```python
from build123d import *

# Parameters (mm, degrees)
SKETCH2_R           = 1.425
BOSS_EXTRUDE1_DEPTH = 3.175


with BuildPart() as part:
    # Sketch2 → Boss-Extrude1 (new body)
    with BuildSketch(Plane(origin=(0, 0, 0), x_dir=(1, 0, 0), z_dir=(0, 1, 0))):
        with BuildLine():
            Line((-145.18277075, -44.880968233), (-179.497120097, -25.768390824))
            ThreePointArc((-179.497120097, -25.768390824), (-183.588653035, -24.128556812), (-187.960968922, -23.569494069))
            Line((-187.960968922, -23.569494069), (-247.377604545, -27.068041697))
            ThreePointArc((-247.377604545, -27.068041697), (-255.760524502, -29.218913898), (-262.07032604, -35.142257782))
            ThreePointArc((-262.07032604, -35.142257782), (-266.807761783, -43.251676507), (-270.933745897, -51.688632391))
            Line((-270.933745897, -51.688632391), (-273.728235609, -57.981701498))
            ThreePointArc((-273.728235609, -57.981701498), (-274.847170355, -61.434035543), (-275.2256366, -65.043382939))
            Line((-275.2256366, -65.043382939), (-275.2256366, -88.130010281))
            ThreePointArc((-275.2256366, -88.130010281), (-270.129294593, -100.433668273), (-257.8256366, -105.530010281))
            Line((-257.8256366, -105.530010281), (-193.494425739, -105.530010281))
            ThreePointArc((-193.494425739, -105.530010281), (-186.835734016, -104.205514146), (-181.190767747, -100.433668273))
            Line((-181.190767747, -100.433668273), (-180.680815133, -99.923715659))
            ThreePointArc((-180.680815133, -99.923715659), (-176.755292612, -97.300765368), (-172.12482308, -96.379707712))
            Line((-172.12482308, -96.379707712), (-153.649556898, -96.379707712))
            ThreePointArc((-153.649556898, -96.379707712), (-141.345898905, -91.283365704), (-136.249556898, -78.979707712))
            Line((-136.249556898, -78.979707712), (-136.249556898, -73.280889471))
            Line((-136.249556898, -73.280889471), (-138.999556898, -73.280889471))
            Line((-138.999556898, -73.280889471), (-138.999556898, -65.780889471))
            Line((-138.999556898, -65.780889471), (-136.249556898, -65.780889471))
            Line((-136.249556898, -65.780889471), (-136.249556898, -60.08207123))
            ThreePointArc((-136.249556898, -60.08207123), (-138.648188978, -51.266235449), (-145.18277075, -44.880968233))
        make_face()
        with Locations(Location((-147.207602145, -91.127288498, 0), (0, 0, 270))):
            Circle(SKETCH2_R, mode=Mode.SUBTRACT)
        with Locations(Location((-141.795027651, -53.115534334, 0), (0, 0, 270))):
            Circle(SKETCH2_R, mode=Mode.SUBTRACT)
        with Locations(Location((-187.963906245, -27.219493821, 0), (0, 0, 270))):
            Circle(SKETCH2_R, mode=Mode.SUBTRACT)
        with Locations(Location((-253.051529835, -31.941972813, 0), (0, 0, 270))):
            Circle(SKETCH2_R, mode=Mode.SUBTRACT)
        with Locations(Location((-267.548354841, -97.852728522, 0), (0, 0, 270))):
            Circle(SKETCH2_R, mode=Mode.SUBTRACT)
        with Locations(Location((-202.85468144, -101.880010281, 0), (0, 0, 270))):
            Circle(SKETCH2_R, mode=Mode.SUBTRACT)
    extrude(amount=BOSS_EXTRUDE1_DEPTH)


solid = part.part
```
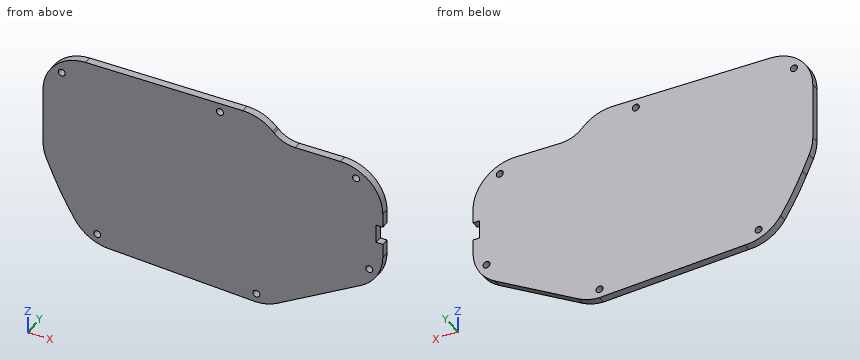
The model under review builds one solid part; all positions refer to its coordinate system, in mm. Round coordinates to 2 decimals unless told otherwise and drop trailing zeros. Loops run counter-clockwise (first coordinate to the right, second up) from the corner with the lowest first, then second, coordinate; pieces in that order, holes last. Notation, with made-up numbers: (89, -32) -> (93, -32) arc R17 cw to (93, -2) -> close; hole circle Ø8 at (87.5, 67.5). An arc over 180 degrees is marked (long way). Answer in a Markdown table with one row per item.
1) Consider section C-C, the plane x = -167.5. Write out the cut boundary in (y, z) (3 decimals), plus the area to 3 significant figures.
Taken from the geometry:
| item | result |
|---|---|
| outline | (0, 32.451) -> (3.175, 32.451) -> (3.175, 96.38) -> (0, 96.38) -> close |
| area | 203 mm² |
2) Consider section A-A, the plane y = 1.25. Count the separate pieces of the cut face and the enclosed holes in it, plus the area to 3 significant figures.
Taken from the geometry:
| item | result |
|---|---|
| separate pieces | 1 |
| enclosed holes | 6 |
| area | 9,640 mm² |
3) Consider section B-B, the plane z = 69.5. Write out the cut boundary in (x, y) (3 decimals).
Taken from the geometry:
| item | result |
|---|---|
| outline | (-275.226, 0) -> (-139, 0) -> (-139, 3.175) -> (-275.226, 3.175) -> close |
4) Wall thickness on line 1 along Z through (x, y) = (-143, 0.7); line 2 along X through (y, z) = (0.55, 52); line 3 along Z through (x, y) = (-247.5, 0.6): over which ranges is each line inside the solid? List them lowest first.
Taken from the geometry:
| item | result |
|---|---|
| line 1 | z = 46.32 to 52.35, 53.88 to 92.74 |
| line 2 | x = -271.07 to -142.68, -140.91 to -138.24 |
| line 3 | z = 27.07 to 105.53 |
5) For pin 1 Ø0.8 at (x, y) = (-137.5, 2) entering from -Z, flat-tipped, find the tip position at first contact; note if it passes through.
Taken from the geometry:
| item | result |
|---|---|
| pin 1 | stops at z = 52.69 |
